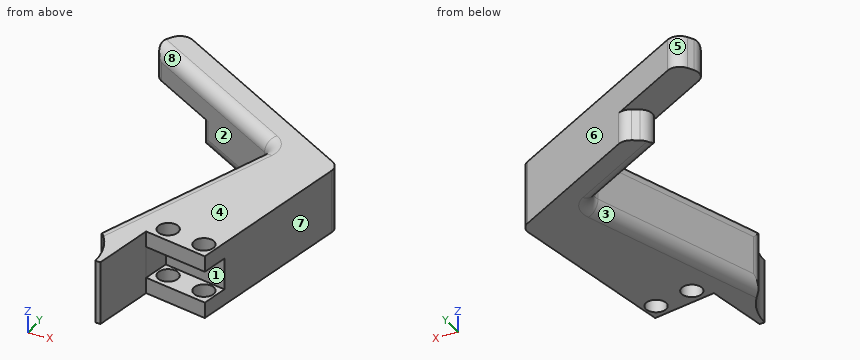
from build123d import *

# Parameters (mm, degrees)
SKETCH3_R           = 2.032
BOSS_EXTRUDE1_DEPTH = 12.7
SKETCH4_W           = 6.35
SKETCH4_H           = 5.498034445
CUT_EXTRUDE1_DEPTH  = 13.0175
CUT_EXTRUDE2_DEPTH  = 6.35
FILLET1_R           = 2.54


with BuildPart() as part:
    # Sketch3 → Boss-Extrude1 (new body)
    with BuildSketch(Plane.XY):
        with BuildLine():
            Line((-70.84525545, 66.890422126), (-58.01103717, 64.713693529))
            Line((-58.01103717, 64.713693529), (-51.782586103, 101.43728904))
            Line((-51.782586103, 101.43728904), (-95.941552678, 126.549550409))
            Line((-95.941552678, 126.549550409), (-99.080585349, 121.029679588))
            Line((-99.080585349, 121.029679588), (-65.256808444, 101.794819897))
            Line((-65.256808444, 101.794819897), (-78.546820512, 64.018247195))
            ThreePointArc((-78.546820512, 64.018247195), (-75.200114259, 59.656734692), (-74.010223155, 54.289482767))
            Line((-74.010223155, 54.289482767), (-72.982419121, 54.289482767))
            Line((-72.982419121, 54.289482767), (-70.84525545, 66.890422126))
        make_face()
        with Locations((-67.846388341, 69.382080978)):
            Circle(SKETCH3_R, mode=Mode.SUBTRACT)
        with Locations((-60.020645487, 68.054807443)):
            Circle(SKETCH3_R, mode=Mode.SUBTRACT)
    extrude(amount=BOSS_EXTRUDE1_DEPTH)

    # Sketch4 → Cut-Extrude1 (cut)
    with BuildSketch(Plane(origin=(-67.057766981, 11.373233325, 0), x_dir=(0, 0, -1), z_dir=(0.98592036, -0.167215563, 0))):
        with Locations((-6.35, 56.851216947)):
            Rectangle(SKETCH4_W, SKETCH4_H)
    extrude(amount=-CUT_EXTRUDE1_DEPTH, mode=Mode.SUBTRACT)

    # Sketch5 → Cut-Extrude2 (cut)
    with BuildSketch(Plane(origin=(0, 0, 0), x_dir=(-1, 0, 0), z_dir=(0, 0, -1))):
        Polygon((99.080585349, 121.029679588), (95.941552678, 126.549550409), (80.927504042, 118.011381544), (87.253435619, 114.30383208), align=None)
    extrude(amount=-CUT_EXTRUDE2_DEPTH, mode=Mode.SUBTRACT)

    # Fillet1
    fillet1_edges = [part.edges().sort_by_distance(p)[0] for p in [
        (-71.901814478, 82.906533546, 0),
        (-76.255122031, 108.049325988, 0),
        (-78.546820512, 64.018247195, 6.35),
        (-65.256808444, 101.794819897, 6.35),
        (-99.080585349, 121.029679588, 9.525),
        (-95.941552678, 126.549550409, 9.525),
        (-51.782586103, 101.43728904, 6.35),
        (-82.168696896, 111.412249742, 12.7),
        (-71.901814478, 82.906533546, 12.7),
        (-87.253435619, 114.30383208, 3.175),
        (-80.927504042, 118.011381544, 3.175),
    ]]
    fillet(fillet1_edges, radius=FILLET1_R)


solid = part.part
Work out the finished part from the listing and answer in its coordinate system (mm). Face numbers are marked on the shaded views. A direction names the side the tool comes from. Coordinates: 2 decimals unless noted, no trailing zeros. Order: outer loops, then holes, each group sorted by start corner. A loop starts at its lowest first (then second) coordinate and runs counter-clockwise, first axis right, second up. Notation, with made-up numbers: (32.5, 68.25) - (88.5, 68.25) arc R8 cw to (88.5, 75.25) - close; hole circle Ø11 at (-16, 88.5). An arc over 180 degrees is marked (long way). Put each result on its own line as item: value. Start each with the question number.
1) Flat-ended cylindrical pins translate along their axes: pin 1 (1 mm diameter, centred on y = 115, z = 2, fed in from +X); pin 2 (1.5 mm diameter, centred on y = 94.5, z = 10, fed in from -X); pin 3 (2.5 mm diameter, centred on x = -61.5, y = 70.5, fed in from -Z); pin 4 (1.5 mm diameter, centred on x = -81.5, z = 4.5, fed in from -Y). Find the tip coordinate at first contact, or state that the pin passes through.
2) Find section D-D (z = 5). Give the vertices of the cut face in (x, y).
3) Find the intervals of material crossed by line 1 (Y direction, x = -58.5, z = 12); line 2 (X direction, y = 100, z = 6.5); line 3 (Y direction, x = -61, z = 7.25), in increasing order. Write a range as from..to.
4) Find section A-A (x = -60.5). Give the vertices of the cut face in (y, z) (3 decimals).
5) For the marked faces 1, 2, 3, 4 and 5, determine the directions among +Z, -Z, +X, -X, +Y, -Y from which every point of the face is accessible in a straight line to the end or side of a thin tool.
6) Find section C-C (x = -69). State how many separate pieces and enclosed holes the cut face has, plus the area to 3 significant figures.
7) For a pull along Y with two mould halves and no side action, classify the marked faces 6, 7 and 8 as released by +Y, released by -Y, zero draft, split by the parting line, or undercut.
8) Find section B-B (z = 11). Give the vertices of the cut face in (x, y), plus the area to 3 significant figures.
Results list:
1. pin 1: stops at x = -74.75
1. pin 2: stops at x = -68.09
1. pin 3: stops at z = 0
1. pin 4: stops at y = 110.61
2. outline: (-83.46, 116.53) arc R2.54 ccw to (-83.43, 112.13) - (-67.1, 102.84) arc R2.54 cw to (-65.96, 99.79) - (-78, 65.57) arc R2.54 ccw to (-77.46, 62.99) arc R12.7 cw to (-74.01, 54.29) - (-72.98, 54.29) - (-69.93, 72.31) - (-57.09, 70.13) - (-52.08, 99.68) arc R2.54 ccw to (-53.33, 102.32) - (-79.65, 117.29) arc R2.54 ccw to (-82.19, 117.27) - close
3. line 1: y = 64.8..66.71, 69.4..105.26
3. line 2: x = -65.9..-52.05
3. line 3: y = 70.8..106.68
4. outline: (65.136, 0) - (66.08, 0) - (66.08, 3.175) - (65.136, 3.175) - close; (65.136, 9.525) - (66.08, 9.525) - (66.08, 12.7) - (65.136, 12.7) - close; (70.029, 0) - (106.395, 0) - (106.395, 12.7) - (70.029, 12.7) - (70.029, 9.525) - (70.712, 9.525) - (70.712, 3.175) - (70.029, 3.175) - close
5. face 1: -Y
5. face 2: +Z, -Z, -X
5. face 3: -Z, -X
5. face 4: +Z, +X, -X, +Y, -Y
5. face 5: +Z, -Z, +Y
6. separate pieces: 4
6. enclosed holes: 0
6. area: 337 mm^2
7. face 6: released by +Y
7. face 7: released by -Y
7. face 8: undercut
8. outline: (-97.82, 123.24) arc R2.54 ccw to (-97.53, 120.31) - (-67.03, 102.97) arc R2.68 cw to (-65.83, 99.75) - (-78.15, 64.73) arc R2.54 ccw to (-77.46, 62.99) arc R12.7 cw to (-74.01, 54.29) - (-72.98, 54.29) - (-70.85, 66.89) - (-58.01, 64.71) - (-52.08, 99.68) arc R2.54 ccw to (-53.33, 102.32) - (-93.73, 125.29) arc R2.54 ccw to (-97.2, 124.34) - close; hole circle Ø4.06 at (-67.85, 69.38); hole circle Ø4.06 at (-60.02, 68.05)
8. area: 892 mm^2
